from build123d import *

# Parameters (mm, degrees)
F0_W     = 101.6
F0_H     = 152.4
F1_DEPTH = 6.35
F2_W     = 63.5
F2_H     = 15.3497201503
F3_DEPTH = 25.4
F4_W     = 101.6
F4_H     = 19.05
F5_DEPTH = 3.96875
F6_W     = 31.75
F6_H     = 31.75
F7_DEPTH = 12.7
F8_W     = 31.75
F8_H     = 31.75
F9_DEPTH = 12.7


# Not quite as in the source:
# - a length typed as a fraction of an inch, garbled in the dataset ("3 / 203.2 mm" for 3/8 in), is restored


with BuildPart() as f1:
    # F0 (on Top) → F1 (new body)
    with BuildSketch(Plane.XY):
        with Locations((50.8, 76.2)):
            Rectangle(F0_W, F0_H)
    extrude(amount=F1_DEPTH)

    # F2 (on face) → F3 (join)
    with BuildSketch(Plane.XY.offset(6.35)):
        with Locations((50.6108440459, 121.0213452578)):
            Rectangle(F2_W, F2_H)
    extrude(amount=F3_DEPTH)

    # F4 (on face) → F5 (join)
    with BuildSketch(Plane.XY.offset(6.35)):
        with Locations((50.8, 142.875)):
            Rectangle(F4_W, F4_H)
    extrude(amount=F5_DEPTH)

    # F6 (on face) → F7 (join)
    with BuildSketch(Plane(origin=(0, 0, 0), x_dir=(1, 0, 0), z_dir=(0, 0, -1))):
        with Locations((15.875, -60.3918848038)):
            Rectangle(F6_W, F6_H)
    extrude(amount=F7_DEPTH)

    # F8 (on face) → F9 (join)
    with BuildSketch(Plane(origin=(0, 0, 0), x_dir=(1, 0, 0), z_dir=(0, 0, -1))):
        with Locations((85.725, -60.325)):
            Rectangle(F8_W, F8_H)
    extrude(amount=F9_DEPTH)


solid = f1.part
CAD build for the part. Positions are in the model's coordinates, mm. A direction names the side the tool comes from. Give positions to 0.01 mm unless a question says otherwise; leave off trailing zeros. Loops run counter-clockwise (first coordinate to the right, second up) from the corner with the lowest first, then second, coordinate; pieces in that order, holes last. Notation, with made-up numbers: M 37,72.5 L 41,72.5 A30 ccw 41,96.5 Z; hole C 32,23 d9. An arc over 180 degrees is marked long. Answer in a Markdown table with one row per item. Add a question column.
Item 1: Band-saw the part on C-C on x = 95.5. Give the cut face in (y, z), then the cut area to 3 significant figures.
Item 2: Probe probe 1 along Z at (x, y) = (35, 45.5); probe 2 along Z at (x, y) = (15.5, 62); probe 3 along X at (y, z) = (75, -3.5). List the from-to ranges inside material, lowest first.
Item 3: Mould opens along Y. For faces 1 (the face through (86, 60, -12.7)), 2 (the face through (50, 133.35, 8)), 3 (the face through (86, 76.2, -6)), 4 (the face through (86, 44.45, -6)) say: +Y half, -Y half, draft (parallel to the pull), parting line (faces both ways), or undercut.
Item 4: Drop flat-ended pins along their axis: P1, Ø12.5, axis at x = 57.5, z = 22, coming from the -Y side; P2, Ø8, axis at x = 23, y = 40, coming from the +Z side; P3, Ø4, axis at x = 91, z = -7.5, coming from the +Y side. Give the stop position or say it passes through.
Item 5: Tool access for faces 5 (the face through (50, 143, 10.319)), 6 (the face through (16, 76.267, -6)), 7 (the face through (31.75, 61, -6)): list every direction of +Z, -Z, +X, -X, +Y, -Y with a clear straight run to the whole face (end or side of a thin tool).
Item 6: Band-saw the part on B-B on y = 118. Give the cut face in (x, z), then the cut area to 3 significant figures.
Item 7: Band-saw the part on A-A on z = -4. Give the cut face in (x, y), then the cut area to 3 significant figures.
Item 8: Band-saw the part on D-D on z = 27.5. Give the cut face in (x, y), then the cut area to 3 significant figures.
Reply:
| question | item | result |
|---|---|---|
| 1 | outline | M 0,0 L 44.45,0 L 44.45,-12.7 L 76.2,-12.7 L 76.2,0 L 152.4,0 L 152.4,10.32 L 133.35,10.32 L 133.35,6.35 L 0,6.35 Z |
| 1 | area | 1,450 mm^2 |
| 2 | probe 1 | z = 0 to 6.35 |
| 2 | probe 2 | z = -12.7 to 6.35 |
| 2 | probe 3 | x = 0 to 31.75, 69.85 to 101.6 |
| 3 | face 1 | draft |
| 3 | face 2 | undercut |
| 3 | face 3 | +Y half |
| 3 | face 4 | -Y half |
| 4 | P1 | stops at y = 113.35 |
| 4 | P2 | stops at z = 6.35 |
| 4 | P3 | stops at y = 76.2 |
| 5 | face 5 | +Z, +X, -X, +Y |
| 5 | face 6 | -Z, +X, -X, +Y |
| 5 | face 7 | -Z, +Y, -Y |
| 6 | outline | M 0,0 L 101.6,0 L 101.6,6.35 L 82.36,6.35 L 82.36,31.75 L 18.86,31.75 L 18.86,6.35 L 0,6.35 Z |
| 6 | area | 2,260 mm^2 |
| 7 | outline | M 0,44.52 L 31.75,44.52 L 31.75,76.27 L 0,76.27 Z; M 69.85,44.45 L 101.6,44.45 L 101.6,76.2 L 69.85,76.2 Z |
| 7 | area | 2,020 mm^2 |
| 8 | outline | M 18.86,113.35 L 82.36,113.35 L 82.36,128.7 L 18.86,128.7 Z |
| 8 | area | 975 mm^2 |
